Answer from the drawing. Dimensions are ordinates in mm from the lowest x, y and z of the part. A direction names the side the tool comes from. Round coordinates to 2 decimals unless told otherwise and drop trailing zeros. Loops run counter-clockwise (first coordinate to the right, second up) from the corner with the lowest first, then second, coordinate; pieces in that order, holes last. Notation, with made-up numbers: (-15, 88.5) - (-9, 88.5) arc R27 cw to (-9, 118.5) - close; hole circle Ø9 at (-29.5, -35). An arc over 180 degrees is marked (long way). Write item = value, one per line. Start each with the question number.
1) For a pull along X with two mould halves and no side action, classify the marked faces 1, 2, 3 and 4 as released by +X, released by -X, zero draft, split by the parting line, or undercut.
2) Section C-C, the plane z = 2 is taken. Determine the outline of the cut face in (x, y), and give its area (3 significant figures).
3) A tool of negligible diameter and unlimited length cuts with its end or side. For the marked faces 5, 6, 7, 8 and 9, from which of +Z, -Z, +X, -X, +Y, -Y can it reach the whole face along a straight path? Write none if from no direction.
4) Section A-A, the plane x = 9 is taken. Determine the outline of the cut face in (y, z), and give its area (3 significant figures).
5) Section D-D, the plane x = 27.5 is taken. Determine the outline of the cut face in (y, z).
6) Given pin 1 Ø11 at (y, z) = (12.5, 14) entering from -X; pin 2 Ø4 at (y, z) = (11.5, 13) entering from +X; pin 3 Ø8.5 at (x, z) = (11.5, 5.5) entering from +Y; pin 4 Ø4 at (x, z) = (8.255, 9.525) entering from +Y, each flat-ended and moving along its own axis, determine where each tip first touches the part or whether it passes through.
7) Section B-B, the plane y = 19 is taken. Determine the outline of the cut face in (x, z).
8) Straight lines are drawn through the part: line 1 along Y through (x, z) = (31.75, 4.25); line 2 along X through (y, z) = (4.5, 10.5); line 3 along Z through (x, y) = (23.5, 26.5). For each, find the intervals that lie inside material, in ascending order.
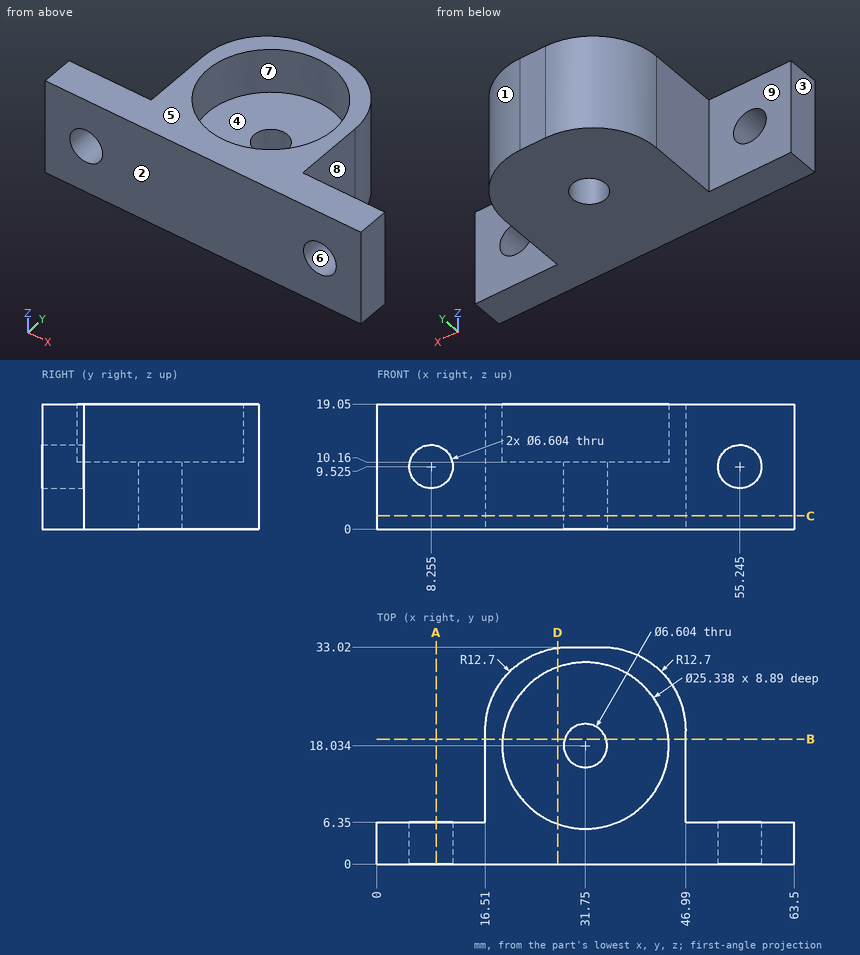
Geometry check:
q1.face_1 = released by +X
q1.face_2 = zero draft
q1.face_3 = released by -X
q1.face_4 = undercut
q2.outline = (0, 0) - (63.5, 0) - (63.5, 6.35) - (46.99, 6.35) - (46.99, 20.32) arc R12.7 ccw to (34.29, 33.02) - (29.21, 33.02) arc R12.7 ccw to (16.51, 20.32) - (16.51, 6.35) - (0, 6.35) - close; hole circle Ø6.6 at (31.75, 18.03)
q2.area = 1,110 mm2
q3.face_5 = +Z, +X, -X, +Y, -Y
q3.face_6 = +Y, -Y
q3.face_7 = +Z
q3.face_8 = +Z, -Z, +X, +Y
q3.face_9 = +Z, -Z, -X, +Y
q4.outline = (0, 0) - (6.35, 0) - (6.35, 6.31) - (0, 6.31) - close; (0, 12.74) - (6.35, 12.74) - (6.35, 19.05) - (0, 19.05) - close
q4.area = 80.1 mm2
q5.outline = (0, 0) - (32.9, 0) - (32.9, 19.05) - (29.97, 19.05) - (29.97, 10.16) - (6.1, 10.16) - (6.1, 19.05) - (0, 19.05) - close
q6.pin_1 = 16.51
q6.pin_2 = 46.99
q6.pin_3 = 6.35
q6.pin_4 = through
q7.outline = (16.51, 0) - (28.59, 0) - (28.59, 10.16) - (19.12, 10.16) - (19.12, 19.05) - (16.51, 19.05) - close; (34.91, 0) - (46.99, 0) - (46.99, 19.05) - (44.38, 19.05) - (44.38, 10.16) - (34.91, 10.16) - close
q8.line_1 = 0 to 14.73, 21.34 to 33.02
q8.line_2 = 0 to 5.1, 11.41 to 52.09, 58.4 to 63.5
q8.line_3 = 0 to 10.16
